Here's how the part is built. I have some questions about the finished solid (model axes, mm). Round coordinates to 2 decimals unless told otherwise and drop trailing zeros. Order: outer loops, then holes, each group sorted by start corner. A loop starts at its lowest first (then second) coordinate and runs counter-clockwise, first axis right, second up. Notation, with made-up numbers: M 3.25,83.5 L 51.25,83.5 A28 ccw 51.25,115.5 Z; hole C 71.5,-19.75 d6. An arc over 180 degrees is marked long. Write item = value, one per line. Start each with the question number.
Item 1: I want a section at A-A, the plane x = -0.4. List the corners of the cut face in (y, z) for me, plus the area to 3 significant figures.
Item 2: I'm going to push flat-ended pins straight in: P1, Ø1.6, axis at x = 0.5, y = 31, coming from the -Z side; P2, Ø1.6, axis at x = 0.5, z = -176, coming from the -Y side; P3, Ø1.6, axis at x = 0.5, z = -174, coming from the +Y side. Where does each tip first touch, or does it pass through?
Item 3: Please list where these lines run through material, in increasing order: L1, parallel to Z at x = -1.2, y = 28; L2, parallel to Y at x = 0.1, z = 168.
```python
from build123d import *

# Parameters (mm, degrees)
SKETCH1_W           = 3.175
SKETCH1_H           = 50.8
BOSS_EXTRUDE1_DEPTH = 191.77
SKETCH1_3_W         = 3.175
SKETCH1_3_H         = 12.7
BOSS_EXTRUDE2_DEPTH = 160.02


with BuildPart() as part:
    # Sketch1 → Boss-Extrude1 (new, symmetric)
    with BuildSketch(Plane.XY):
        Rectangle(SKETCH1_W, SKETCH1_H)
    extrude(amount=BOSS_EXTRUDE1_DEPTH, both=True)

    # Sketch1<3> → Boss-Extrude2 (add, symmetric)
    with BuildSketch(Plane.XY):
        with Locations((0, 31.75)):
            Rectangle(SKETCH1_3_W, SKETCH1_3_H)
        with Locations((0, -31.75)):
            Rectangle(SKETCH1_3_W, SKETCH1_3_H)
    extrude(amount=BOSS_EXTRUDE2_DEPTH, both=True)


solid = part.part
```
Filled in:
q1.outline = M -38.1,-160.02 L -25.4,-160.02 L -25.4,-191.77 L 25.4,-191.77 L 25.4,-160.02 L 38.1,-160.02 L 38.1,160.02 L 25.4,160.02 L 25.4,191.77 L -25.4,191.77 L -25.4,160.02 L -38.1,160.02 Z
q1.area = 27,600 mm^2
q2.P1 = -160.02
q2.P2 = -25.4
q2.P3 = 25.4
q3.L1 = -160.02 to 160.02
q3.L2 = -25.4 to 25.4
